Print and shaded views of the part. All mm, measured from the part's lowest x, y and z. A direction names the side the tool comes from. Round coordinates to 2 decimals unless told otherwise and drop trailing zeros. Write each loop counter-clockwise with the first axis right and the second up, starting at its lowest first coordinate (ties: lowest second). Pieces come first, ordered by that corner, then holes. Notation, with made-up numbers: M 11.5,24.25 L 50.5,24.25 A16 cw 50.5,38.25 Z; hole C 69,61.5 d4. An arc over 180 degrees is marked long. Write item = value, one per line. Start each with the question number.
Q1. Band-saw the part on D-D on x = 36.5. Write the cut outline in (y, z), plus the area to 4 significant figures.
Q2. Pull direction Y, two halves, no side cores. Call the marked faces 1, 2 and 3: released by +Y, released by -Y, zero draft, split by the parting line, or undercut.
Q3. Tool access for the marked faces 4, 5 and 6: list every direction of +Z, -Z, +X, -X, +Y, -Y with a clear straight run to the whole face (end or side of a thin tool).
Q4. Band-saw the part on A-A on z = 7.25. Write the cut outline in (x, y), plus the area to 3 significant figures.
Q5. Band-saw the part on C-C on y = 20.5. Write the cut outline in (x, z), plus the area to 3 significant figures.
Q6. Drop flat-ended pins along their axis: P1, Ø1.2, axis at y = 7, z = 2, coming from the -X side; P2, Ø2, axis at y = 27.5, z = 6.5, coming from the +X side; P3, Ø13, axis at x = 30, y = 11, coming from the +Z side. Give the stop position or say it passes through.
Q7. Probe L1, parallel to Y at x = 10.5, z = 4.25; L2, parallel to Y at x = 16, z = 7; L3, parallel to X at y = 5.25, z = 1.25. List the from-to ranges inside material, lowest first.
Q8. Band-saw the part on B-B on x = 50.5. Write the cut outline in (y, z), plus the area to 4 significant figures.
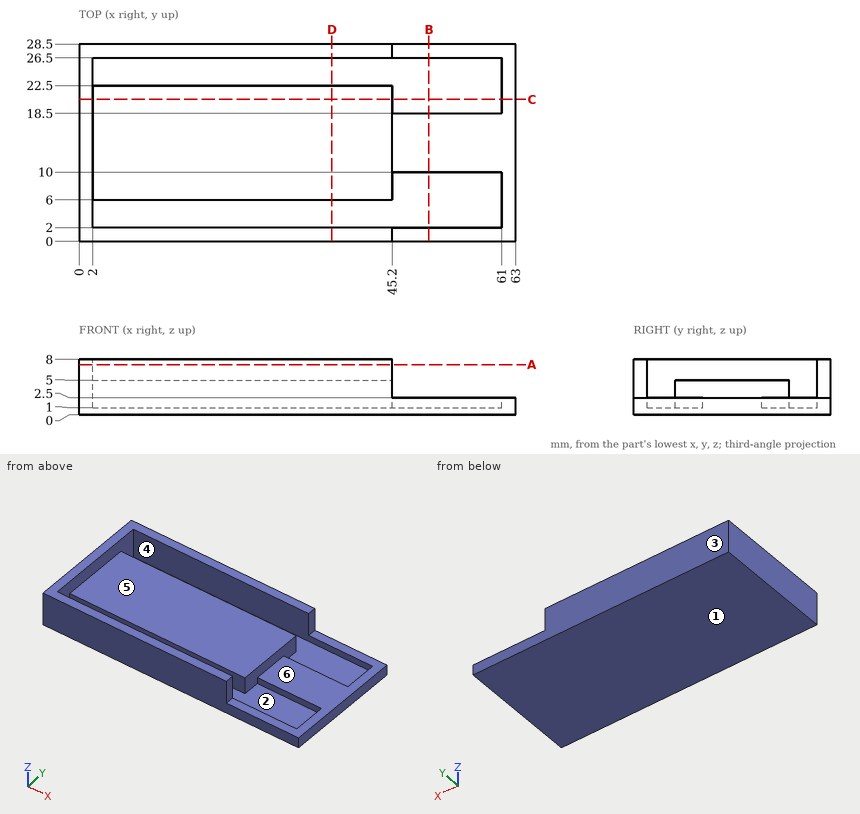
Conclusion:
q1.outline = M 0,0 L 28.5,0 L 28.5,8 L 26.5,8 L 26.5,1 L 22.5,1 L 22.5,5 L 6,5 L 6,1 L 2,1 L 2,8 L 0,8 Z
q1.area = 122.5 mm^2
q2.face_1 = zero draft
q2.face_2 = undercut
q2.face_3 = released by +Y
q3.face_4 = +Z
q3.face_5 = +Z, +X
q3.face_6 = +Z, +X, +Y, -Y
q4.outline = M 0,0 L 45.2,0 L 45.2,2 L 2,2 L 2,26.5 L 45.2,26.5 L 45.2,28.5 L 0,28.5 Z
q4.area = 230 mm^2
q5.outline = M 0,0 L 63,0 L 63,2.5 L 61,2.5 L 61,1 L 45.2,1 L 45.2,5 L 2,5 L 2,8 L 0,8 Z
q5.area = 253 mm^2
q6.P1 = 0
q6.P2 = 45.2
q6.P3 = 5
q7.L1 = 0 to 2, 6 to 22.5, 26.5 to 28.5
q7.L2 = 0 to 2, 26.5 to 28.5
q7.L3 = 0 to 2, 61 to 63
q8.outline = M 0,0 L 28.5,0 L 28.5,2.5 L 26.5,2.5 L 26.5,1 L 18.5,1 L 18.5,2.5 L 10,2.5 L 10,1 L 2,1 L 2,2.5 L 0,2.5 Z
q8.area = 47.25 mm^2
